Answer from the drawing. Dimensions are ordinates in mm from the lowest x, y and z of the part. Coordinates: 2 decimals unless noted, no trailing zeros. Put each result on its own line as item: value.
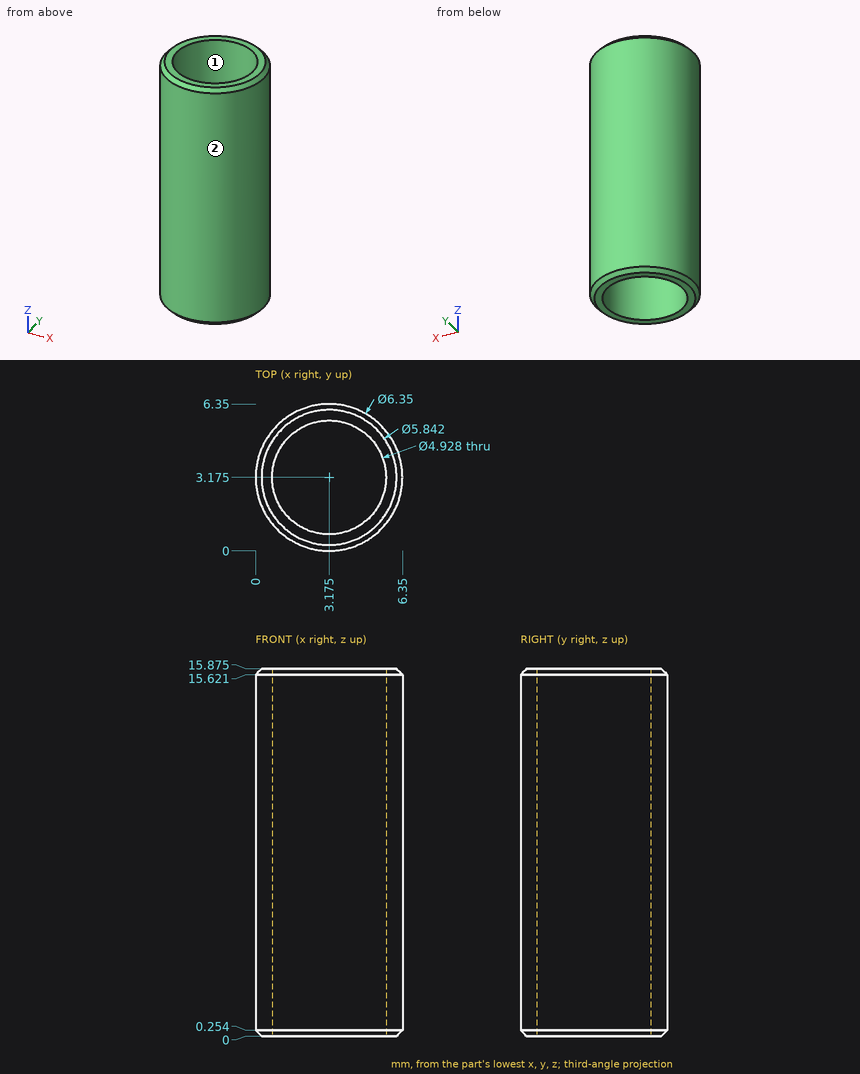
1) Straight lines are drawn through the part: line 1 (X direction, y = 4, z = 1.5); line 2 (X direction, y = 5, z = 2) (1 decimal). For each, find the intervals that lie inside material, in ascending order. Write a range as [from, to].
Answer list:
line 1: x = [0.11, 0.85], [5.5, 6.24]
line 2: x = [0.6, 1.5], [4.8, 5.8]
2) Given pin 1 Ø1 at (y, z) = (4, 2) entering from -X, flat-ended and moving along its own axis, determine where the tip first touches the part or whether it passes through.
Answer list:
pin 1: stops at x = 0.02
3) Determine the mould class of the marked faces 1 and 2 for opening direction Y: released by +Y, released by -Y, zero draft, split by the parting line, or undercut.
Answer list:
face 1: undercut
face 2: split by the parting line
